Autodesk Inventor part; units mm, degrees
ref_plane "YZ Plane" through (0, 0, 0) normal (1, 0, 0) x (0, 1, 0)
ref_plane "XZ Plane" through (0, 0, 0) normal (0, 1, 0) x (-1, 0, 0)
ref_plane "XY Plane" through (0, 0, 0) normal (0, 0, 1) x (1, 0, 0)
sketch "Skizze1" plane through (0, 0, 0) normal (0, 0, 1) x (1, 0, 0)
  line L0 (-24, 0) -> (144, 0)
  line L1 (0, -27) -> (0, 162)
  line L2 (0, 0) -> (120, 0)
  line L3 (120, 0) -> (120, 135)
  line L4 (120, 135) -> (0, 135)
  line L5 (0, 135) -> (0, 0)
  point P0 (0, 135)
  dimension "d0" = 135
  dimension "d1" = 120
extrude "Extrusion1" add sketch "Skizze1" along normal blind 10
sketch "Skizze2" plane through (0, 0, 10) normal (0, 0, 1) x (1, 0, 0)
  line L0 (0, 0) -> (120, 0)
  line L1 (33, 0) -> (87, 0)
  line L2 (87, 0) -> (87, 25)
  line L3 (87, 25) -> (33, 25)
  line L4 (33, 25) -> (33, 0)
  line L5 (0, 135) -> (0, 0)
  dimension "d4" = 54
  dimension "d5" = 25
  dimension "d6" = 33
extrude "Extrusion2" cut sketch "Skizze2" against normal blind 5
sketch "Skizze3" plane through (0, 0, 0) normal (0, 0, -1) x (-1, 0, 0)
  line L0 (-75, 115) -> (-70, 115)
  line L1 (-70, 115) -> (-70, 110)
  line L2 (-70, 110) -> (-75, 110)
  line L3 (-75, 110) -> (-75, 115)
  line L4 (-50, 115) -> (-45, 115)
  line L5 (-45, 115) -> (-45, 110)
  line L6 (-45, 110) -> (-50, 110)
  line L7 (-50, 110) -> (-50, 115)
  line L8 (-120, 135) -> (0, 135)
  line L9 (-120, 0) -> (-120, 135)
  line L10 (0, 135) -> (0, 0)
  line L11 (-120, 135) -> (0, 135)
  dimension "d9" = 5
  dimension "d10" = 5
  dimension "d11" = 5
  dimension "d12" = 5
  dimension "d13" = 20
  dimension "d14" = 20
  dimension "d15" = 45
  dimension "d16" = 45
  dimension "d17" = 20
extrude "Extrusion3" add sketch "Skizze3" along normal blind 20
sketch "Skizze4" plane through (75, 110, 0) normal (1, 0, 0) x (0, 0, -1)
  line L0 (0, 5) -> (20, 5)
  line L1 (20, 5) -> (25, 5)
  line L2 (25, 5) -> (25, 0)
  line L3 (25, 0) -> (20, 0)
  line L4 (20, 0) -> (20, 5)
  point P0 (0, -110)
  dimension "d20" = 5
  dimension "d21" = 5
extrude "Extrusion4" add sketch "Skizze4" against normal blind 30
fillet "Rundung1" radius 2.5 12 edges at (60, 110, -25) (60, 115, -25) (75, 115, -12.5) (75, 110, -12.5) (45, 110, -12.5) (50, 110, -10) (70, 110, -10) (60, 110, -20) (50, 115, -10) (60, 115, -20) (70, 115, -10) (45, 115, -12.5)
properties part number "DeckelMess_Better" material "Acetalharz, Schwarz"
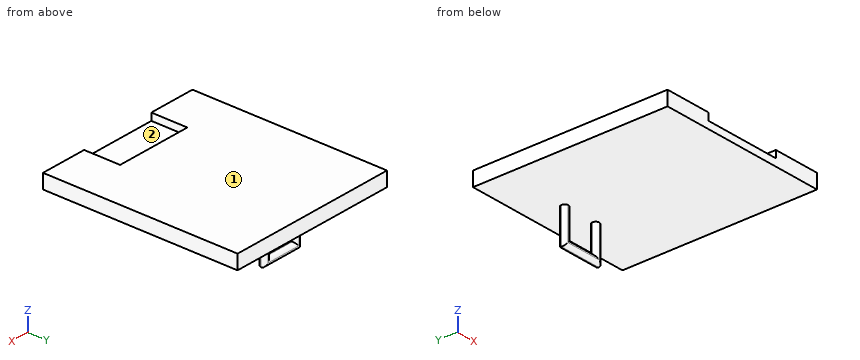
Source: CAD feature listing. Evaluate the final solid. Frame: model axes, mm. Face numbers are marked on the shaded views. Give positions to 0.01 mm unless a question says otherwise; leave off trailing zeros. Loops run counter-clockwise (first coordinate to the right, second up) from the corner with the lowest first, then second, coordinate; pieces in that order, holes last. Notation, with made-up numbers: (14, -39.5) -> (51, -39.5) arc R31 cw to (51, -8.5) -> close; hole circle Ø1 at (21, -23.5). An arc over 180 degrees is marked (long way). Use a Markdown table: item, result. Add a question column.
(1) Ray query, line 1 (Z direction, x = 56, y = 47); line 2 (Z direction, x = 77.5, y = 12); line 3 (Y direction, x = 70.5, z = -23). Return the intervals inside material, ascending.
(2) Pull-direction query (X, two-part tool) for the marked faces 1 and 2; classes: +X half, -X half, draft (parallel to the pull), parting line (faces both ways), or undercut.
(3) Section query C-C (y = 16). Output: boundary loops of the cut face in (x, z).
(4) First-contact query: pin 1 Ø4 at (y, z) = (9, 7.5) entering from -X; pin 2 Ø11.5 at (x, z) = (54, -14.5) entering from -Y; pin 3 Ø4 at (x, y) = (46, 14.5) entering from +Z; pin 4 Ø3 at (x, y) = (88, 77) entering from -Z. Flat tips, straight axial feed; report the tip coordinate or a pass-through.
(5) Section query D-D (x = 79). Output: boundary loops of the cut face in (y, z), then the cut area to 4 significant figures.
Checked values:
| question | item | result |
|---|---|---|
| 1 | line 1 | 0 to 10 |
| 1 | line 2 | 0 to 5 |
| 1 | line 3 | 110.05 to 114.95 |
| 2 | face 1 | draft |
| 2 | face 2 | undercut |
| 3 | outline | (0, 0) -> (120, 0) -> (120, 10) -> (87, 10) -> (87, 5) -> (33, 5) -> (33, 10) -> (0, 10) -> close |
| 4 | pin 1 | x = 0 |
| 4 | pin 2 | y = 110.12 |
| 4 | pin 3 | z = 5 |
| 4 | pin 4 | z = 0 |
| 5 | outline | (0, 0) -> (135, 0) -> (135, 10) -> (25, 10) -> (25, 5) -> (0, 5) -> close |
| 5 | area | 1,225 mm^2 |
